The listing builds one solid part. Answer for the finished solid, in the listing's coordinates (mm). A direction names the side the tool comes from. Round coordinates to 2 decimals unless told otherwise and drop trailing zeros. Order: outer loops, then holes, each group sorted by start corner. A loop starts at its lowest first (then second) coordinate and runs counter-clockwise, first axis right, second up. Notation, with made-up numbers: (-5.75, -36.75) -> (13.25, -36.75) arc R26 ccw to (13.25, -4.75) -> close; hole circle Ø2 at (40, -6). An arc over 180 degrees is marked (long way). Answer in a Markdown table with one row per item. Add a question column.
Autodesk Inventor part; units mm, degrees
ref_plane "YZ Plane" through (0, 0, 0) normal (1, 0, 0) x (0, 1, 0)
ref_plane "XZ Plane" through (0, 0, 0) normal (0, 1, 0) x (-1, 0, 0)
ref_plane "XY Plane" through (0, 0, 0) normal (0, 0, 1) x (1, 0, 0)
sketch "Sketch1" plane through (0, 0, 0) normal (0, 1, 0) x (-1, 0, 0)
  line L0 (0, 0) -> (-24, 0)
  line L1 (-24, -48) -> (0, -48)
  line L2 (0, -48) -> (0, 0)
  circle A0 centre (-12, -33) radius 2
  circle A1 centre (-12, -18) radius 2
  line L3 (-24, -48) -> (-38, -48)
  line L4 (-38, -48) -> (-38, -24)
  line L5 (-38, -24) -> (-24, -24)
  line L6 (-24, -27) -> (-24, -45)
  line L7 (-24, -45) -> (-35, -45)
  line L8 (-35, -45) -> (-35, -27)
  line L9 (-35, -27) -> (-24, -27)
  line L10 (-24, -27) -> (-24, -45)
  line L11 (-24, 0) -> (-24, -24)
  line L12 (-24, -27) -> (-24, -45)
  line L13 (-28.5, -45) -> (-30.5, -45)
  line L14 (-30.5, -45) -> (-30.5, -27)
  line L15 (-30.5, -27) -> (-28.5, -27)
  line L16 (-28.5, -27) -> (-28.5, -45)
  point P0 (-12, -48)
  dimension "d0" = 24
  dimension "d1" = 48
  dimension "d2" = 4
  dimension "d3" = 4
  dimension "d4" = 15
  dimension "d5" = 30
  dimension "d6" = 14
  dimension "d7" = 24
  dimension "d8" = 3
  dimension "d9" = 3
  dimension "d10" = 3
  dimension "d11" = 48
  dimension "d12" = 11
  dimension "d27" = 18
  dimension "d28" = 4.5
  dimension "d29" = 4.5
extrude "Extrusion1" add sketch "Sketch1" along normal blind 6 contours L2 L1 L3 L4 L5 L11 L0 | L16 L7 L14 L9
sketch "Sketch2" plane through (0, 6, 0) normal (0, 1, 0) x (1, 0, 0)
  line L0 (2, 48) -> (22, 48)
  line L1 (22, 48) -> (22, 0)
  line L2 (22, 0) -> (2, 0)
  line L3 (2, 0) -> (2, 48)
  line L4 (0, 0) -> (24, 0)
  point P0 (12, 0)
  point P1 (12, 0)
  dimension "d15" = 20
  dimension "d16" = 48
extrude "Extrusion2" cut sketch "Sketch2" against normal blind 1
sketch "Sketch3" plane through (38, 0, -24) normal (1, 0, 0) x (0, 0, -1)
  circle A0 centre (12, 3) radius 1.5
  line L0 (24, 0) -> (24, 6)
  line L1 (0, 6) -> (24, 6)
  point P0 (-24, 0)
  point P1 (24, 3)
  point P2 (12, 6)
  dimension "d19" = 3
extrude "Extrusion3" cut sketch "Sketch3" against normal through all
sketch "Sketch4" plane through (24, 0, 0) normal (1, 0, 0) x (0, 0, -1)
  circle A0 centre (12, 3) radius 1.5
  line L0 (0, 0) -> (0, 6)
  point P0 (0, 3)
  dimension "d22" = 3
  dimension "d23" = 12
extrude "Extrusion4" cut sketch "Sketch4" against normal through all
sketch "Sketch5" plane through (24, 0, -27) normal (1, 0, 0) x (0, 0, -1)
  circle A0 centre (9, 3) radius 1.5
  circle A1 centre (9, 3) radius 1.5
  circle A2 centre (9, 3) radius 2
  point P0 (-27, 0)
  dimension "d30" = 3
  dimension "d31" = 4
extrude "Extrusion5" add sketch "Sketch5" along normal blind 12
sketch "Sketch6" plane through (0, 6, 0) normal (0, 1, 0) x (1, 0, 0)
  line L0 (30.75, 42.7686) -> (34.75, 42.7686)
  line L1 (34.75, 42.7686) -> (34.75, 30.7686)
  line L2 (34.75, 30.7686) -> (30.75, 30.7686)
  line L3 (30.75, 30.7686) -> (30.75, 42.7686)
  line L4 (30.5, 27) -> (30.5, 45)
  line L5 (24.25, 42.1188) -> (28.25, 42.1188)
  line L6 (28.25, 42.1188) -> (28.25, 30.1188)
  line L7 (28.25, 30.1188) -> (24.25, 30.1188)
  line L8 (24.25, 30.1188) -> (24.25, 42.1188)
  line L9 (24, 27) -> (24, 45)
  point P0 (0, 0)
  dimension "d34" = 4
  dimension "d35" = 12
  dimension "d36" = 0.25
  dimension "d37" = 4
  dimension "d38" = 12
  dimension "d39" = 0.25
extrude "Extrusion6" cut sketch "Sketch6" against normal through all
fillet "Fillet1" radius 12 1 edges at (24, 3, -24)
fillet "Fillet2" radius 2 3 edges at (38, 3, -24) (38, 3, -48) (0, 3, -48)
properties part number "rightshortNEW1"
1. Each of these flat-tipped pins is pushed along its axis until it touches: pin 1 (3.5 mm diameter, centred on x = 12, z = -33, fed in from +Y); pin 2 (5 mm diameter, centred on x = 12, z = -18, fed in from +Y). Where does it stop, or does it pass through?
2. The mould has two halves that part along Y. Classify faces 4 (the cylindrical face through (36.4, 2.1, -34.8)), 5 (the flat face through (12, 3, 0)), 6 (the flat face through (15, 0, -24)), 7 (the cylindrical face through (12.2, 2.1, -10.8)): released by +Y, released by -Y, zero draft, split by the parting line, or undercut.
3. For faces 1 (the flat face through (24, 3, -6)), 2 (the flat face through (22, 5.5, -24.3)), 3 (the flat face through (38, 1, -36)), determine the directions among +Z, -Z, +X, -X, +Y, -Y from which every point of the face is accessible in a straight line to the end or side of a thin tool.
4. The part is cut by section A-A (z = -27.5). Give the vertices of the cut face in (x, y), then the cut area to 3 significant figures.
5. The part is cut by section B-B (y = 5.5). Give the number of separate pieces and of enclosed holes in the cut face, then the cut area to 3 significant figures.
6. The part is cut by section D-D (x = 17.5). Give the vertices of the cut face in (y, z), then the cut area to 3 significant figures.
7. The part is cut by section C-C (z = -33). Give the vertices of the cut face in (x, y).
8. Straight lines are drawn through the part: line 1 along Z through (x, y) = (15.5, 3); line 2 along X through (y, z) = (3.15, -33); line 3 along X through (y, z) = (4, -28). For each, find the intervals that lie inside material, in ascending order.
Report:
| question | item | result |
|---|---|---|
| 1 | pin 1 | passes through |
| 1 | pin 2 | stops at y = 5 |
| 2 | face 4 | undercut |
| 2 | face 5 | zero draft |
| 2 | face 6 | released by -Y |
| 2 | face 7 | undercut |
| 3 | face 1 | +Z, +X, +Y, -Y |
| 3 | face 2 | +Z, -Z, +Y |
| 3 | face 3 | +Z, -Z, +X, +Y, -Y |
| 4 | outline | (0, 0) -> (24, 0) -> (24, 6) -> (22, 6) -> (22, 5) -> (2, 5) -> (2, 6) -> (0, 6) -> close; (28.5, 0) -> (30.5, 0) -> (30.5, 6) -> (28.5, 6) -> close; (35, 0) -> (38, 0) -> (38, 6) -> (35, 6) -> close |
| 4 | area | 154 mm^2 |
| 5 | separate pieces | 2 |
| 5 | enclosed holes | 2 |
| 5 | area | 394 mm^2 |
| 6 | outline | (0, -48) -> (5, -48) -> (5, 0) -> (0, 0) -> close; hole circle Ø3 at (3, -36); hole circle Ø3 at (3, -12) |
| 6 | area | 226 mm^2 |
| 7 | outline | (0, 0) -> (10, 0) -> (10, 5) -> (2, 5) -> (2, 6) -> (0, 6) -> close; (14, 0) -> (24, 0) -> (24, 6) -> (22, 6) -> (22, 5) -> (14, 5) -> close; (28.5, 0) -> (30.5, 0) -> (30.5, 6) -> (28.5, 6) -> close; (35, 0) -> (38, 0) -> (38, 6) -> (35, 6) -> close |
| 8 | line 1 | z = -48 to -37.5, -34.5 to -13.5, -10.5 to 0 |
| 8 | line 2 | x = 0 to 10, 14 to 24, 28.5 to 30.5, 35 to 38 |
| 8 | line 3 | x = 0 to 24, 28.5 to 30.5, 35 to 38 |
